Read the model definition and answer for the solid it produces. Units are mm, in the model's axes. A direction names the side the tool comes from. Round coordinates to 2 decimals unless told otherwise and drop trailing zeros. Loops run counter-clockwise (first coordinate to the right, second up) from the corner with the lowest first, then second, coordinate; pieces in that order, holes last. Notation, with made-up numbers: M -8.5,-39 L 0.5,-39 A6 ccw 0.5,-29 Z; hole C 13.5,52 d7. An arc over 180 degrees is marked long. Write each question's results on one line, items separated by ' | '.
```python
from build123d import *

# Parameters (mm, degrees)
BOSS_EXTRUDE1_DEPTH = 10.15
CUT_EXTRUDE1_DEPTH  = 20.3


with BuildPart() as part:
    # Sketch1 → Boss-Extrude1 (new, symmetric)
    with BuildSketch(Plane(origin=(0, 0, 0), x_dir=(1, 0, 0), z_dir=(0, 1, 0))):
        Polygon((0, 0), (0, -27.5), (27.5, 0), align=None)
    extrude(amount=BOSS_EXTRUDE1_DEPTH, both=True)

    # Sketch2 → Cut-Extrude1 (cut)
    with BuildSketch(Plane.ZY):
        with BuildLine():
            Line((15, -2.5), (10, -2.5))
            ThreePointArc((10, -2.5), (7.5, 0), (10, 2.5))
            Line((10, 2.5), (15, 2.5))
            ThreePointArc((15, 2.5), (17.5, 0), (15, -2.5))
        make_face()
    extrude(amount=-CUT_EXTRUDE1_DEPTH, mode=Mode.SUBTRACT)


solid = part.part
```
1. Find section B-B, the plane y = 0. Give the vertices of the cut face in (x, z).
Completed:
outline: M 0,0 L 27.5,0 L 20,7.5 L 0,7.5 Z; M 0,17.5 L 10,17.5 L 0,27.5 Z
2. Determine the mould class of faces 3 (the face through (13.6, -4.4, 13.9)), 4 (the face through (11, 10.15, 11)), 5 (the face through (7, 2.5, 12)), 6 (the face through (14, 0, 0)) for opening direction Z: released by +Z, released by -Z, zero draft, split by the parting line, or undercut.
Completed:
face 3: released by +Z | face 4: zero draft | face 5: undercut | face 6: released by -Z
3. Given P1, Ø6, axis at x = 20.5, y = 1, coming from the +Z side; P2, Ø1, axis at y = -3.5, z = 9.5, coming from the +X side; P3, Ø2, axis at x = 24, z = 5, coming from the +Y side, each flat-ended and moving along its own axis, determine where each tip first touches the part or whether it passes through.
Completed:
P1: stops at z = 9.62 | P2: stops at x = 18.5 | P3: passes through
4. Find section D-D, the plane x = 15.25. Give the vertices of the cut face in (y, z), then the cut area to 3 significant figures.
Completed:
outline: M -10.15,0 L 10.15,0 L 10.15,12.25 L 2.5,12.25 L 2.5,10 A2.5 cw -2.5,10 L -2.5,12.25 L -10.15,12.25 Z | area: 228 mm2
5. Find section C-C, the plane x = 6.5. Give the vertices of the cut face in (y, z).
Completed:
outline: M -10.15,0 L 10.15,0 L 10.15,21 L -10.15,21 Z; hole M -2.5,10 A2.5 ccw 2.5,10 L 2.5,15 A2.5 ccw -2.5,15 Z
6. Find section A-A, the plane z = 14. Give the vertices of the cut face in (x, y).
Completed:
outline: M 0,-10.15 L 13.5,-10.15 L 13.5,-2.5 L 0,-2.5 Z; M 0,2.5 L 13.5,2.5 L 13.5,10.15 L 0,10.15 Z
7. Find the intervals of material crossed by L1, parallel to Y at x = 3.25, z = 10.5; L2, parallel to X at y = -0.75, z = 20; L3, parallel to Z at x = 6.25, y = -0.5, in increasing order.
Completed:
L1: y = -10.15 to -2.5, 2.5 to 10.15 | L2: x = 0 to 7.5 | L3: z = 0 to 7.55, 17.45 to 21.25
8. Which of the six approach directions +Z, -Z, +X, -X, +Y, -Y give full straight-line access (tool end or side, diameter ignored) to faces 1 (the face through (0, 2, 17)), 2 (the face through (4.8, 0.1, 17.5))?
Completed:
face 1: +Z, -Z, -X, +Y, -Y | face 2: +X, -X
